Work out the finished part from the listing and answer in its coordinate system (mm). Face numbers are marked on the shaded views. A direction names the side the tool comes from. Give positions to 0.01 mm unless a question says otherwise; leave off trailing zeros. Loops run counter-clockwise (first coordinate to the right, second up) from the corner with the lowest first, then second, coordinate; pieces in that order, holes last. Notation, with made-up numbers: M 79.25,69 L 128.25,69 A25 ccw 128.25,86 Z; hole C -6,-11.75 d2. An arc over 180 degrees is marked long. Write item = value, one per line. Start each with the question number.
1. Consider L1, parallel to Y at x = 0, z = 6; L2, parallel to Y at x = -9.5, z = 6.25; L3, parallel to Y at x = 7, z = 7. Determine where each line is inside the solid, lowest interval first. Write a range as [from, to].
2. Flat-ended cylindrical pins translate along their axes: pin 1 Ø8 at (x, y) = (-9, -11.5) entering from +Z; pin 2 Ø6.5 at (x, y) = (-10.7, 3.48) entering from -Z; pin 3 Ø8 at (y, z) = (-1, 10) entering from +X; pin 4 Ø2.5 at (x, z) = (-1, 8.5) entering from -Y. Find the tip coordinate at first contact, or state that the pin passes through.
3. For the marked faces 1, 2 and 3, determine the directions among +Z, -Z, +X, -X, +Y, -Y from which every point of the face is accessible in a straight line to the end or side of a thin tool.
4. Section A-A on x = 0 is taken. Give the number of separate pieces and of enclosed holes in the cut face, plus the area to 3 significant figures.
5. The mould has two halves that part along Z. Classify the marked faces 4, 5 and 6: released by +Z, released by -Z, zero draft, split by the parting line, or undercut.
6. Section C-C on z = 9.75 is taken. Determine the outline of the cut face in (x, y).
7. Section B-B on y = -8.5 is taken. Determine the outline of the cut face in (x, z).
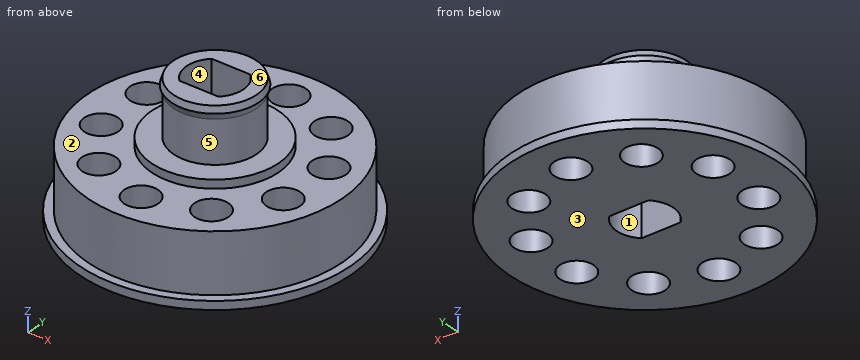
```python
from build123d import *

# Parameters (mm, degrees)
F3_R      = 15
F3_R_2    = 2
F3_R_3    = 7.5
F3_R_4    = 4.9
F4_DEPTH  = 8
F5_DEPTH  = 9
F6_DEPTH  = 15.5
F3_R_5    = 16
F11_DEPTH = 1


with BuildPart() as f4:
    # F3 (on Top) → F4 (new body)
    with BuildSketch(Plane.XY):
        Circle(F3_R)
        with Locations((-6.6125840883, -9.1014411867)):
            Circle(F3_R_2, mode=Mode.SUBTRACT)
        with Locations((-10.6993858083, -3.4764411867)):
            Circle(F3_R_2, mode=Mode.SUBTRACT)
        with Locations((0, -11.25)):
            Circle(F3_R_2, mode=Mode.SUBTRACT)
        with Locations((6.6125840883, -9.1014411867)):
            Circle(F3_R_2, mode=Mode.SUBTRACT)
        with Locations((10.6993858083, -3.4764411867)):
            Circle(F3_R_2, mode=Mode.SUBTRACT)
        with Locations((-10.6993858083, 3.4764411867)):
            Circle(F3_R_2, mode=Mode.SUBTRACT)
        with Locations((-6.6125840883, 9.1014411867)):
            Circle(F3_R_2, mode=Mode.SUBTRACT)
        Circle(F3_R_3, mode=Mode.SUBTRACT)
        with Locations((10.6993858083, 3.4764411867)):
            Circle(F3_R_2, mode=Mode.SUBTRACT)
        with Locations((0, 11.25)):
            Circle(F3_R_2, mode=Mode.SUBTRACT)
        with Locations((6.6125840883, 9.1014411867)):
            Circle(F3_R_2, mode=Mode.SUBTRACT)
        Circle(F3_R_3)
        Circle(F3_R_4, mode=Mode.SUBTRACT)
        Circle(F3_R_4)
        with BuildLine():
            ThreePointArc((-2.2847319318, -2.45), (-3.35, 0), (-2.2847319318, 2.45))
            Line((-2.2847319318, 2.45), (2.2847319318, 2.45))
            ThreePointArc((2.2847319318, 2.45), (3.35, 0), (2.2847319318, -2.45))
            Line((2.2847319318, -2.45), (-2.2847319318, -2.45))
        make_face(mode=Mode.SUBTRACT)
    extrude(amount=F4_DEPTH)

    # F3 (on Top) → F5 (join)
    with BuildSketch(Plane.XY):
        Circle(F3_R_3)
        Circle(F3_R_4, mode=Mode.SUBTRACT)
        Circle(F3_R_4)
        with BuildLine():
            ThreePointArc((-2.2847319318, -2.45), (-3.35, 0), (-2.2847319318, 2.45))
            Line((-2.2847319318, 2.45), (2.2847319318, 2.45))
            ThreePointArc((2.2847319318, 2.45), (3.35, 0), (2.2847319318, -2.45))
            Line((2.2847319318, -2.45), (-2.2847319318, -2.45))
        make_face(mode=Mode.SUBTRACT)
    extrude(amount=F5_DEPTH)

    # F3 (on Top) → F6 (join)
    with BuildSketch(Plane.XY):
        Circle(F3_R_4)
        with BuildLine():
            ThreePointArc((-2.2847319318, -2.45), (-3.35, 0), (-2.2847319318, 2.45))
            Line((-2.2847319318, 2.45), (2.2847319318, 2.45))
            ThreePointArc((2.2847319318, 2.45), (3.35, 0), (2.2847319318, -2.45))
            Line((2.2847319318, -2.45), (-2.2847319318, -2.45))
        make_face(mode=Mode.SUBTRACT)
    extrude(amount=F6_DEPTH)

    # F7 (on Front) → F8 (revolve)
    with BuildSketch(Plane.XZ):
        Polygon((5.15, 14.75), (4.9, 15.5), (4.9, 14), align=None)
    revolve(axis=Axis((0, 0, 8.7542282417), (0, 0, 1)))

    # F3 (on Top) → F11 (join)
    with BuildSketch(Plane.XY):
        Circle(F3_R_5)
        Circle(F3_R, mode=Mode.SUBTRACT)
    extrude(amount=F11_DEPTH)


solid = f4.part
```
Verdict:
q1.L1 = [-15, -13.25], [-9.25, -2.45], [2.45, 9.25], [13.25, 15]
q1.L2 = [-11.61, -5.08], [-1.88, 1.88], [5.08, 11.61]
q1.L3 = [-13.27, -11.06], [-7.14, 7.14], [11.06, 13.27]
q2.pin_1 = 8
q2.pin_2 = 0
q2.pin_3 = 15
q2.pin_4 = -15
q3.face_1 = +Z, -Z
q3.face_2 = +Z
q3.face_3 = -Z, +X, -X, +Y, -Y
q4.separate_pieces = 4
q4.enclosed_holes = 0
q4.area = 181 mm2
q5.face_4 = zero draft
q5.face_5 = undercut
q5.face_6 = released by +Z
q6.outline = C 0,0 d9.8; hole M -2.28,-2.45 L 2.28,-2.45 A3.35 ccw 2.28,2.45 L -2.28,2.45 A3.35 ccw Z
q7.outline = M -13.56,0 L -8.52,0 L -8.52,8 L -12.36,8 L -12.36,1 L -13.56,1 Z; M -4.71,0 L 4.71,0 L 4.71,8 L -4.71,8 Z; M 8.52,0 L 13.56,0 L 13.56,1 L 12.36,1 L 12.36,8 L 8.52,8 Z
